from build123d import *

# Parameters (mm, degrees)
SKETCH1_R           = 5
SKETCH1_R_2         = 0.75
BOSS_EXTRUDE1_DEPTH = 3


with BuildPart() as part:
    # Sketch1 → Boss-Extrude1 (new body)
    with BuildSketch(Plane.XY):
        Polygon((-13.25, 15.5), (-10.25, 15.5), (-10.25, 10.5), (-13.25, 10.5), (-13.25, 5.35), (-10.25, 5.35), (-10.25, 0.35), (-13.25, 0.35), (-13.25, -4.65), (-10.25, -4.65), (-10.25, -9.65), (-13.25, -9.65), (-13.25, -20.5), (13.25, -20.5), (13.25, -9.65), (10.25, -9.65), (10.25, -4.65), (13.25, -4.65), (13.25, 0.35), (10.25, 0.35), (10.25, 5.35), (13.25, 5.35), (13.25, 10.5), (10.25, 10.5), (10.25, 15.5), (13.25, 15.5), (13.25, 20.5), (13.25, 26.25), (-13.25, 26.25), (-13.25, 20.5), align=None)
        with Locations((0, 16.54)):
            Circle(SKETCH1_R, mode=Mode.SUBTRACT)
        with Locations((0, 24.04)):
            Circle(SKETCH1_R_2, mode=Mode.SUBTRACT)
        with Locations((6.495302374, 20.289806272)):
            Circle(SKETCH1_R_2, mode=Mode.SUBTRACT)
        with Locations((6.495190528, 12.79)):
            Circle(SKETCH1_R_2, mode=Mode.SUBTRACT)
        with Locations((0, 9.04)):
            Circle(SKETCH1_R_2, mode=Mode.SUBTRACT)
        with Locations((-6.495302374, 12.790193728)):
            Circle(SKETCH1_R_2, mode=Mode.SUBTRACT)
        with Locations((-6.495190528, 20.29)):
            Circle(SKETCH1_R_2, mode=Mode.SUBTRACT)
    extrude(amount=BOSS_EXTRUDE1_DEPTH)


solid = part.part
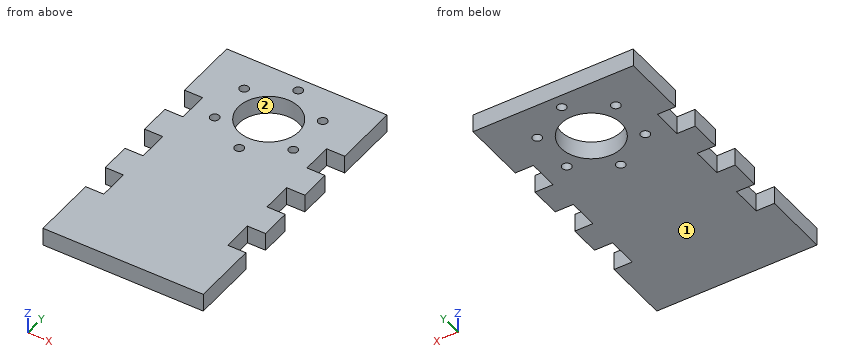
Part model, mm, in its own coordinate system. Face numbers are marked on the shaded views. Round coordinates to 2 decimals unless told otherwise and drop trailing zeros. Write each loop counter-clockwise with the first axis right and the second up, starting at its lowest first coordinate (ties: lowest second). Pieces come first, ordered by that corner, then holes. Notation, with made-up numbers: M 69,-34 L 89,-34 A27 ccw 89,1 Z; hole C -34.5,87 d2. An arc over 180 degrees is marked long. Return JSON: item names as keys, results as strings. Group by question number.
(1) Saw through at D-D on z = 1.2. Count the separate pieces of the cut face and the enclosed holes in it, then the cut area to 3 significant figures.
(2) Saw through at B-B on y = 24.04. Write the cut outline in (x, z), then the cut area to 3 significant figures.
(3) Drill centre lines: probe 1 along Y at (x, z) = (-10.5, 1.2); probe 2 along Y at (x, z) = (0, 1.8); probe 3 along Y at (x, z) = (6.5, 1.75). Where is each one in solid material? Low to high.
(4) Saw through at A-A on x = 0. Write the cut outline in (y, z).
(5) Pin check, flat tips, straight feed: pin 1 Ø1.5 at (y, z) = (4, 2) entering from -X; pin 2 Ø1.5 at (y, z) = (-8, 1.5) entering from +X. Stop position of each tip, or through.
(6) Saw through at C-C on y = 16.54. Write the cut outline in (x, z).
(7) Two-plate mould, pull along Y, no slides. Class the marked faces 1 and 2: +Y half, -Y half, draft (parallel to the pull), parting line (faces both ways), or undercut.
Returned:
{
 "1": {"separate pieces": "1", "enclosed holes": "7", "area": "1,060 mm²"},
 "2": {"outline": "M -13.25,0 L -0.75,0 L -0.75,3 L -13.25,3 Z; M 0.75,0 L 13.25,0 L 13.25,3 L 0.75,3 Z", "area": "75.0 mm²"},
 "3": {"probe 1": "-20.5 to -9.65, -4.65 to 0.35, 5.35 to 10.5, 15.5 to 26.25", "probe 2": "-20.5 to 8.29, 9.79 to 11.54, 21.54 to 23.29, 24.79 to 26.25", "probe 3": "-20.5 to 12.04, 13.54 to 19.54, 21.04 to 26.25"},
 "4": {"outline": "M -20.5,0 L 8.29,0 L 8.29,3 L -20.5,3 Z; M 9.79,0 L 11.54,0 L 11.54,3 L 9.79,3 Z; M 21.54,0 L 23.29,0 L 23.29,3 L 21.54,3 Z; M 24.79,0 L 26.25,0 L 26.25,3 L 24.79,3 Z"},
 "5": {"pin 1": "x = -10.25", "pin 2": "x = 10.25"},
 "6": {"outline": "M -13.25,0 L -5,0 L -5,3 L -13.25,3 Z; M 5,0 L 13.25,0 L 13.25,3 L 5,3 Z"},
 "7": {"face 1": "draft", "face 2": "undercut"}
}
